from build123d import *

# Parameters (mm, degrees)
F0_R     = 4.99
F1_DEPTH = 45
F2_R     = 5.5454073787
F2_R_2   = 4.99
F3_DEPTH = 2
F4_R     = 4.5
F5_DEPTH = 1
F6_R     = 4.99
F6_R_2   = 4.5
F7_DEPTH = 1.5


with BuildPart() as f1:
    # F0 (on Right) → F1 (new body)
    with BuildSketch(Plane.YZ):
        Circle(F0_R)
    extrude(amount=F1_DEPTH)

    # F2 (on face) → F3 (join)
    with BuildSketch(Plane(origin=(0, 0, 0), x_dir=(0, -1, 0), z_dir=(-1, 0, 0))):
        Circle(F2_R)
        Circle(F2_R_2, mode=Mode.SUBTRACT)
        Circle(F2_R_2)
    extrude(amount=F3_DEPTH)

    # F4 (on face) → F5 (join)
    with BuildSketch(Plane.YZ.offset(45)):
        Circle(F4_R)
    extrude(amount=F5_DEPTH)

    # F6 (on face) → F7 (join)
    with BuildSketch(Plane.YZ.offset(46)):
        Circle(F6_R)
        Circle(F6_R_2, mode=Mode.SUBTRACT)
        Circle(F6_R_2)
    extrude(amount=F7_DEPTH)


solid = f1.part
For this review, take the finished solid that the model builds, in its own axes (mm). A direction names the side the tool comes from. Round coordinates to 2 decimals unless told otherwise and drop trailing zeros. Loops run counter-clockwise (first coordinate to the right, second up) from the corner with the lowest first, then second, coordinate; pieces in that order, holes last. Notation, with made-up numbers: (53, 89.25) - (77, 89.25) arc R22 ccw to (77, 124.25) - close; hole circle Ø5 at (64.5, -4.75). An arc over 180 degrees is marked (long way). Use one line per item in the form item = value.
1) We need section A-A on y = 0. Write out the cut boundary in (x, z), then the cut area to 3 significant figures.
Solutions:
outline = (-2, -5.55) - (0, -5.55) - (0, -4.99) - (45, -4.99) - (45, -4.5) - (46, -4.5) - (46, -4.99) - (47.5, -4.99) - (47.5, 4.99) - (46, 4.99) - (46, 4.5) - (45, 4.5) - (45, 4.99) - (0, 4.99) - (0, 5.55) - (-2, 5.55) - close
area = 495 mm2
2) Clearance check with flat-ended pins moving along their axes: P1, Ø5, axis at x = 12, y = 1.5, coming from the -Z side; P2, Ø6, axis at x = 38, z = -2, coming from the -Y side; P3, Ø3, axis at x = 24.5, z = -2.5, coming from the -Y side. State where each tip first meets the part, or that it passes through.
Solutions:
P1 = -4.99
P2 = -4.99
P3 = -4.89
3) Wall thickness on probe 1 along X at (y, z) = (1, 4.5); probe 2 along X at (y, z) = (-0.5, -5); probe 3 along Z at (x, y) = (5, -0.25): over which ranges is each line inside the solid? List them lowest first.
Solutions:
probe_1 = -2 to 45, 46 to 47.5
probe_2 = -2 to 0
probe_3 = -4.98 to 4.98
4) We need section C-C on x = 20.5. Write out the cut boundary in (y, z).
Solutions:
outline = circle Ø9.98 at (0, 0)
5) Mouldability with a two-part tool opening along X and no side actions: class faces 3 (the face through (0, 5, 2)), 4 (the face through (46.74, -0.65, 4.948)), 5 (the face through (-2, 0, 0)), 6 (the face through (45.49, -0.59, 4.46)) as pulls with the +X half, pulls with the -X half, needs draft (parallel to the pull), parting line crosses it, or undercut.
Solutions:
face_3 = pulls with the +X half
face_4 = needs draft
face_5 = pulls with the -X half
face_6 = undercut
6) Tool access review of faces 1 (the face through (-0.99, -5.29, 1.67)), 2 (the face through (22.185, -0.65, 4.948)): name each direction out of +Z, -Z, +X, -X, +Y, -Y from which nothing blocks a thin tool from reaching the whole face with its end or side.
Solutions:
face_1 = +X, -X
face_2 = +X
